The listing builds one solid part. Answer for the finished solid, in the listing's coordinates (mm). A direction names the side the tool comes from. Round coordinates to 2 decimals unless told otherwise and drop trailing zeros. Write each loop counter-clockwise with the first axis right and the second up, starting at its lowest first coordinate (ties: lowest second). Pieces come first, ordered by that corner, then holes. Notation, with made-up numbers: (55.25, 38.25) - (90.25, 38.25) arc R13 cw to (90.25, 50.25) - close; hole circle Ø10 at (43, 33). An arc over 180 degrees is marked (long way). Return JSON: item names as keys, results as strings. Group by question number.
(1) Section A-A, the plane x = 10.5 is taken. Write down the section's boundary in (y, z), then the cut area to 3 significant figures.
(2) Section B-B, the plane z = 7 is taken. Write down the section's boundary in (x, y), then the cut area to 3 significant figures.
(3) Section C-C, the plane y = -5 is taken. Write down the section's boundary in (x, z) (3 decimals).
(4) Each of these flat-tipped pins is pushed along its axis until it touches: pin 1 (8 mm diameter, centred on y = 4.5, z = -2, fed in from -X); pin 2 (4 mm diameter, centred on y = -5.5, z = -4.5, fed in from -X); pin 3 (1.4 mm diameter, centred on x = 3, y = -1, fed in from +Z). Where does it stop, or does it pass through?
(5) Find the intervals of material crossed by line 1 along Y through (x, z) = (0.25, 3); line 2 along Y through (x, z) = (-0.75, -6.5); line 3 along Z through (x, y) = (12, -2.25), in increasing order. Write a range as [from, to].
(6) Which of the six approach directions +Z, -Z, +X, -X, +Y, -Y give full straight-line access (tool end or side, diameter ignored) to faces 1 (the cylindrical face through (15, -3, 0)), 2 (the flat face through (2, 0, -3.24)), 3 (the flat face through (2, -3.24, 0)), 4 (the flat face through (2, 0, 3.24)), 5 (the flat face through (2, 3.24, 0))?
```python
from build123d import *

# Parameters (mm, degrees)
CUT_REVOLVE_1_2_OUTLINE_W = 6.48
CUT_REVOLVE_1_2_OUTLINE_H = 6.48
CUT_REVOLVE_1_2_DEPTH     = 4.6


with BuildPart() as part:
    # 草图1 → Revolve 699 (revolve)
    with BuildSketch(Plane.XY):
        with BuildLine():
            Line((-1.081081081, 8), (0, 8))
            Line((0, 8), (0, 0))
            Line((0, 0), (-3.6, 0))
            ThreePointArc((-3.6, 0), (-2.955391275, 4.193594893), (-1.081081081, 8))
        make_face()
    revolve(axis=Axis((-3.6, 0, 0), (1, 0, 0)))



with BuildPart() as body_2:
    # 切除-旋转1: read off the stored shape, not the designer's step
    # 切除-旋转1 outline → 切除-旋转1 (revolve)
    with BuildSketch(Plane.YX):
        Polygon((3, 24.500014667), (2.134, 25), (0, 25), (0, 4.240398306), (3, 4.240398306), align=None)
    revolve(axis=Axis((0, 0, 0), (1, 0, 0)))


with BuildPart() as part_1:
    add(part.part)

    add(body_2.part)  # Cut-Revolve 1 2 merges body 2
    # Cut-Revolve 1 2 outline → Cut-Revolve 1 2 (add)
    with BuildSketch(Plane.YZ):
        Rectangle(CUT_REVOLVE_1_2_OUTLINE_W, CUT_REVOLVE_1_2_OUTLINE_H)
    extrude(amount=CUT_REVOLVE_1_2_DEPTH)

    # Cut-Revolve 1 3 outline → Cut-Revolve 1 3 (revolve, cut)
    with BuildSketch(Plane.YX):
        Polygon((4.582051794, 4.6), (3.24, 4.6), (4.582051794, 4.240398306), align=None)
    revolve(axis=Axis((0, 0, 0), (1, 0, 0)), mode=Mode.SUBTRACT)


solid = part_1.part
```
Working result:
{
 "1": {"outline": "circle Ø6 at (0, 0)", "area": "28.3 mm^2"},
 "2": {"outline": "(-1.08, -3.87) - (0, -3.87) - (0, 3.87) - (-1.08, 3.87) arc R12.08 ccw to start", "area": "11.7 mm^2"},
 "3": {"outline": "(-1.081, -6.245) - (0, -6.245) - (0, 6.245) - (-1.081, 6.245) arc R13.037 ccw to start"},
 "4": {"pin 1": "stops at x = -3.57", "pin 2": "stops at x = -2.63", "pin 3": "stops at z = 3.24"},
 "5": {"line 1": "y = [-3.24, 3.24]", "line 2": "y = [-4.66, 4.66]", "line 3": "z = [-1.98, 1.98]"},
 "6": {"face 1": "+X", "face 2": "-Z, +X, +Y, -Y", "face 3": "+Z, -Z, +X, -Y", "face 4": "+Z, +X, +Y, -Y", "face 5": "+Z, -Z, +X, +Y"}
}
